Can you work these out from the model? Positions are in its coordinate system, mm. A direction names the side the tool comes from. Round coordinates to 2 decimals unless told otherwise and drop trailing zeros. Write each loop counter-clockwise with the first axis right and the second up, starting at its lowest first coordinate (ties: lowest second). Pieces come first, ordered by that corner, then holes.
Q1. If we section it at B-B (y = -175): Please give me the cut outline in (x, z).
Q2. If we section it at A-A (z = 2): Please give me the cut outline in (x, y).
Q3. I'm going to push flat-ended pins straight in: pin 1 Ø3 at (x, z) = (34.5, 9) entering from +Y; pin 2 Ø5 at (x, y) = (18.5, -250) entering from +Z; pin 3 Ø6.5 at (y, z) = (-129, 4.5) entering from +X. Where does each tip first touch, or does it pass through?
Q4. For faces 5 (the flat face through (19, -175, 0)), 6 (the flat face through (3, -140.208, 6)), 7 (the flat face through (35, -114.808, 6)), which set-ups out of +Z, -Z, +X, -X, +Y, -Y let a thin tool reach every point of the face, with its end or its side?
Q5. Please list where these lines run through material, in increasing order: line 1 along Y through (x, z) = (32.5, 1.25); line 2 along X through (y, z) = (-314.5, 11.25); line 3 along X through (y, z) = (-135.5, 7).
Q6. We'd pull the mould along X, two halves only. Please class faces 1 (the flat face through (19, 0, 6)), 2 (the flat face through (3, -114.808, 6)), 3 (the flat face through (19, -175, 11.176)), 4 (the flat face through (31.496, -128, 6)): +X half, -X half, draft (parallel to the pull), parting line (faces both ways), or undercut.
from build123d import *

# Parameters (mm, degrees)
F1_DEPTH = 355.6
F2_W     = 25.4
F2_H     = 12.7
F3_DEPTH = 6.35


# Not quite as in the source:
# - a pattern or mirror of a feature is missing from the dataset's text; its kind, count and spacing are read off the source's solid


with BuildPart() as f1:
    # F0 (on Front) → F1 (new body)
    with BuildSketch(Plane.XZ):
        Polygon((15.748, 12.7), (0, 12.7), (0, 0), (37.846, 0), (37.846, 12.7), (22.098, 12.7), (22.098, 11.176), (15.748, 11.176), align=None)
    extrude(amount=F1_DEPTH)

    # F2 (on face) → F3 (cut)
    with BuildSketch(Plane.YZ.offset(37.846)):
        with Locations((-127.508, 6.35)):
            Rectangle(F2_W, F2_H)
    f3 = extrude(amount=-F3_DEPTH, mode=Mode.SUBTRACT)

    # F3_copies: F3 across plane
    add(f3.mirror(Plane(origin=(19.05, 0, 0), x_dir=(0, 0, -1), z_dir=(-1, 0, 0))), mode=Mode.SUBTRACT)


solid = f1.part
A:
1. outline: (0, 0) - (37.85, 0) - (37.85, 12.7) - (22.1, 12.7) - (22.1, 11.18) - (15.75, 11.18) - (15.75, 12.7) - (0, 12.7) - close
2. outline: (0, -355.6) - (37.85, -355.6) - (37.85, -140.21) - (31.5, -140.21) - (31.5, -114.81) - (37.85, -114.81) - (37.85, 0) - (0, 0) - close; hole (0.25, -140.21) - (6.6, -140.21) - (6.6, -114.81) - (0.25, -114.81) - close
3. pin 1: stops at y = 0
3. pin 2: stops at z = 11.18
3. pin 3: stops at x = 31.5
4. face 5: -Z, +X, -X, +Y, -Y
4. face 6: +Z, -Z
4. face 7: +Z, -Z, +X
5. line 1: y = -355.6 to -140.21, -114.81 to 0
5. line 2: x = 0 to 15.75, 22.1 to 37.85
5. line 3: x = 0 to 0.25, 6.6 to 31.5
6. face 1: draft
6. face 2: undercut
6. face 3: undercut
6. face 4: +X half
